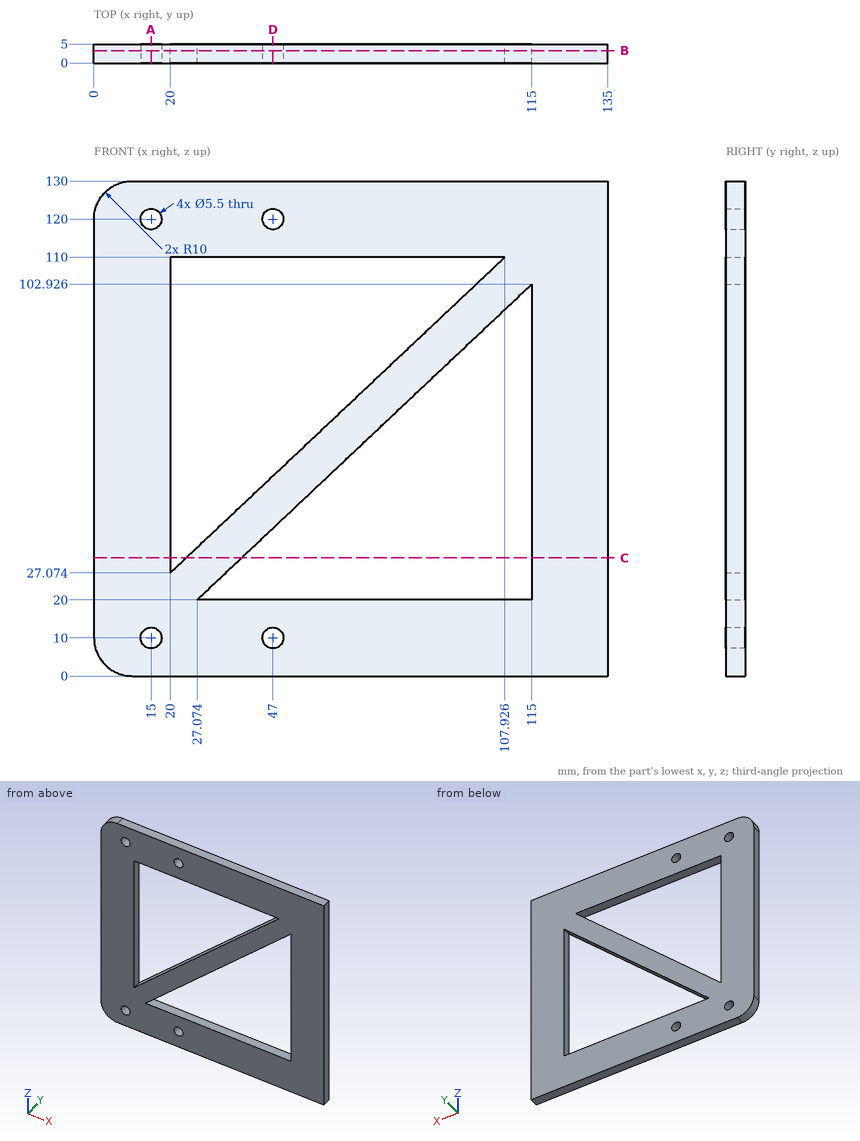
The drawing under review shows one solid part. Ordinate dimensions are in mm from its lowest x, y, z. Coordinates: 2 decimals unless noted, no trailing zeros. Write each loop counter-clockwise with the first axis right and the second up, starting at its lowest first coordinate (ties: lowest second). Pieces come first, ordered by that corner, then holes. Notation, with made-up numbers: (-27.75, 56.5) - (20.25, 56.5) arc R16 ccw to (20.25, 72.5) - close; hole circle Ø4 at (87, 6.5). An arc over 180 degrees is marked (long way). Answer in a Markdown table with one row per item. Add a question column.
Q1. We need section C-C, the plane z = 31. State the section outline as (x, y) points.
Q2. We need section A-A, the plane x = 15. State the section outline as (y, z) points, and give its area (3 significant figures).
Q3. We need section D-D, the plane x = 47. State the section outline as (y, z) points, and give its area (3 significant figures).
Q4. For probe 1 along X at (y, z) = (3.7, 120); probe 2 along Z at (x, y) = (71, 2.85); probe 3 along Z at (x, y) = (101, 2), list the stretches that pass through material, from the lowest coordinate up.
Q5. For P1, Ø4.5, axis at x = 47, z = 10, coming from the -Y side, flat-tipped, find the tip position at first contact; note if it passes through.
Q6. We need section B-B, the plane y = 3.25. State the section outline as (x, z) points, and give its area (3 significant figures).
Answer list:
| question | item | result |
|---|---|---|
| 1 | outline | (0, 0) - (20, 0) - (20, 5) - (0, 5) - close; (24.16, 0) - (38.74, 0) - (38.74, 5) - (24.16, 5) - close; (115, 0) - (135, 0) - (135, 5) - (115, 5) - close |
| 2 | outline | (0, 0) - (5, 0) - (5, 7.25) - (0, 7.25) - close; (0, 12.75) - (5, 12.75) - (5, 117.25) - (0, 117.25) - close; (0, 122.75) - (5, 122.75) - (5, 130) - (0, 130) - close |
| 2 | area | 595 mm2 |
| 3 | outline | (0, 0) - (5, 0) - (5, 7.25) - (0, 7.25) - close; (0, 12.75) - (5, 12.75) - (5, 20) - (0, 20) - close; (0, 38.79) - (5, 38.79) - (5, 52.54) - (0, 52.54) - close; (0, 110) - (5, 110) - (5, 117.25) - (0, 117.25) - close; (0, 122.75) - (5, 122.75) - (5, 130) - (0, 130) - close |
| 3 | area | 214 mm2 |
| 4 | probe 1 | x = 0 to 12.25, 17.75 to 44.25, 49.75 to 135 |
| 4 | probe 2 | z = 0 to 20, 61.43 to 75.17, 110 to 130 |
| 4 | probe 3 | z = 0 to 20, 89.72 to 103.47, 110 to 130 |
| 5 | P1 | passes through |
| 6 | outline | (0, 10) arc R10 ccw to (10, 0) - (135, 0) - (135, 130) - (10, 130) arc R10 ccw to (0, 120) - close; hole circle Ø5.5 at (15, 10); hole circle Ø5.5 at (15, 120); hole (20, 27.07) - (107.93, 110) - (20, 110) - close; hole (27.07, 20) - (115, 20) - (115, 102.93) - close; hole circle Ø5.5 at (47, 10); hole circle Ø5.5 at (47, 120) |
| 6 | area | 10,100 mm2 |
